```python
from build123d import *

# Parameters (mm, degrees)
SKETCH1_W                      = 203.2
SKETCH1_H                      = 203.2
BOSS_EXTRUDE1_DEPTH            = 76.2
SKETCH2_W                      = 196.85
SKETCH2_H                      = 196.85
CUT_EXTRUDE1_DEPTH             = 73.025
CUT_EXTRUDE2_REACH             = 241.623
SKETCH3_R                      = 4.7625
SKETCH3_R_2                    = 3.175
SKETCH3_W                      = 19.05
SKETCH3_H                      = 19.05
CUT_EXTRUDE2_DIRECTION_2_DEPTH = 240.623120754
CUT_EXTRUDE3_REACH             = 241.623
SKETCH4_R                      = 3.175
SKETCH4_W                      = 25.4
SKETCH4_H                      = 9.525
CUT_EXTRUDE4_REACH             = 241.623
SKETCH5_W                      = 25.4
SKETCH5_H                      = 9.525


with BuildPart() as part:
    # Sketch1 → Boss-Extrude1 (new body)
    with BuildSketch(Plane(origin=(0, 0, 0), x_dir=(1, 0, 0), z_dir=(0, 1, 0))):
        Rectangle(SKETCH1_W, SKETCH1_H)
    extrude(amount=BOSS_EXTRUDE1_DEPTH)

    # Sketch2 → Cut-Extrude1 (cut)
    with BuildSketch(Plane(origin=(0, 76.2, 0), x_dir=(1, 0, 0), z_dir=(0, 1, 0))):
        Rectangle(SKETCH2_W, SKETCH2_H)
    extrude(amount=-CUT_EXTRUDE1_DEPTH, mode=Mode.SUBTRACT)

    # Sketch3 → Cut-Extrude2 (cut, up to next)
    with BuildSketch(Plane(origin=(101.6, 0, 0), x_dir=(0, 0, -1), z_dir=(1, 0, 0)), mode=Mode.PRIVATE) as cut_extrude2_sk1:
        with Locations(Location((-69.85, 12.7, 0), (0, 0, 180))):
            Circle(SKETCH3_R)
    cut_extrude2_tool1 = extrude(cut_extrude2_sk1.sketch, amount=-CUT_EXTRUDE2_REACH, mode=Mode.PRIVATE) & part.part
    # Sketch3 → Cut-Extrude2 (cut, up to next)
    with BuildSketch(Plane(origin=(101.6, 0, 0), x_dir=(0, 0, -1), z_dir=(1, 0, 0)), mode=Mode.PRIVATE) as cut_extrude2_sk2:
        with Locations(Location((-57.15, 12.7, 0), (0, 0, 180))):
            Circle(SKETCH3_R)
    cut_extrude2_tool2 = extrude(cut_extrude2_sk2.sketch, amount=-CUT_EXTRUDE2_REACH, mode=Mode.PRIVATE) & part.part
    # Sketch3 → Cut-Extrude2 (cut, up to next)
    with BuildSketch(Plane(origin=(101.6, 0, 0), x_dir=(0, 0, -1), z_dir=(1, 0, 0)), mode=Mode.PRIVATE) as cut_extrude2_sk3:
        with Locations(Location((-44.45, 12.7, 0), (0, 0, 180))):
            Circle(SKETCH3_R)
    cut_extrude2_tool3 = extrude(cut_extrude2_sk3.sketch, amount=-CUT_EXTRUDE2_REACH, mode=Mode.PRIVATE) & part.part
    # Sketch3 → Cut-Extrude2 (cut, up to next)
    with BuildSketch(Plane(origin=(101.6, 0, 0), x_dir=(0, 0, -1), z_dir=(1, 0, 0)), mode=Mode.PRIVATE) as cut_extrude2_sk4:
        with Locations(Location((-31.75, 12.7, 0), (0, 0, 180))):
            Circle(SKETCH3_R)
    cut_extrude2_tool4 = extrude(cut_extrude2_sk4.sketch, amount=-CUT_EXTRUDE2_REACH, mode=Mode.PRIVATE) & part.part
    # Sketch3 → Cut-Extrude2 (cut, up to next)
    with BuildSketch(Plane(origin=(101.6, 0, 0), x_dir=(0, 0, -1), z_dir=(1, 0, 0)), mode=Mode.PRIVATE) as cut_extrude2_sk5:
        with Locations(Location((-88.9, 63.5, 0), (0, 0, 180))):
            Circle(SKETCH3_R_2)
    cut_extrude2_tool5 = extrude(cut_extrude2_sk5.sketch, amount=-CUT_EXTRUDE2_REACH, mode=Mode.PRIVATE) & part.part
    # Sketch3 → Cut-Extrude2 (cut, up to next)
    with BuildSketch(Plane(origin=(101.6, 0, 0), x_dir=(0, 0, -1), z_dir=(1, 0, 0)), mode=Mode.PRIVATE) as cut_extrude2_sk6:
        with Locations((22.225, 12.7)):
            Rectangle(SKETCH3_W, SKETCH3_H)
    cut_extrude2_tool6 = extrude(cut_extrude2_sk6.sketch, amount=-CUT_EXTRUDE2_REACH, mode=Mode.PRIVATE) & part.part
    add(cut_extrude2_tool1.solids().sort_by_distance((101.6, 12.7, 69.85))[0], mode=Mode.SUBTRACT)
    add(cut_extrude2_tool2.solids().sort_by_distance((101.6, 12.7, 57.15))[0], mode=Mode.SUBTRACT)
    add(cut_extrude2_tool3.solids().sort_by_distance((101.6, 12.7, 44.45))[0], mode=Mode.SUBTRACT)
    add(cut_extrude2_tool4.solids().sort_by_distance((101.6, 12.7, 31.75))[0], mode=Mode.SUBTRACT)
    add(cut_extrude2_tool5.solids().sort_by_distance((101.6, 63.5, 88.9))[0], mode=Mode.SUBTRACT)
    add(cut_extrude2_tool6.solids().sort_by_distance((101.6, 12.7, -22.225))[0], mode=Mode.SUBTRACT)

    # Sketch3 → Cut-Extrude2 direction 2 (cut)
    with BuildSketch(Plane(origin=(101.6, 0, 0), x_dir=(0, 0, -1), z_dir=(1, 0, 0))):
        with Locations(Location((-69.85, 12.7, 0), (0, 0, 180))):
            Circle(SKETCH3_R)
        with Locations(Location((-57.15, 12.7, 0), (0, 0, 180))):
            Circle(SKETCH3_R)
        with Locations(Location((-44.45, 12.7, 0), (0, 0, 180))):
            Circle(SKETCH3_R)
        with Locations(Location((-31.75, 12.7, 0), (0, 0, 180))):
            Circle(SKETCH3_R)
        with Locations(Location((-88.9, 63.5, 0), (0, 0, 180))):
            Circle(SKETCH3_R_2)
        with Locations((22.225, 12.7)):
            Rectangle(SKETCH3_W, SKETCH3_H)
    extrude(amount=CUT_EXTRUDE2_DIRECTION_2_DEPTH, mode=Mode.SUBTRACT)

    # Sketch4 → Cut-Extrude3 (cut, up to next)
    with BuildSketch(Plane(origin=(0, 0, -101.6), x_dir=(-1, 0, 0), z_dir=(0, 0, -1)), mode=Mode.PRIVATE) as cut_extrude3_sk1:
        with Locations((0, 38.1)):
            Circle(SKETCH4_R)
    cut_extrude3_tool1 = extrude(cut_extrude3_sk1.sketch, amount=-CUT_EXTRUDE3_REACH, mode=Mode.PRIVATE) & part.part
    # Sketch4 → Cut-Extrude3 (cut, up to next)
    with BuildSketch(Plane(origin=(0, 0, -101.6), x_dir=(-1, 0, 0), z_dir=(0, 0, -1)), mode=Mode.PRIVATE) as cut_extrude3_sk2:
        with Locations((50.8, 38.1)):
            Rectangle(SKETCH4_W, SKETCH4_H)
    cut_extrude3_tool2 = extrude(cut_extrude3_sk2.sketch, amount=-CUT_EXTRUDE3_REACH, mode=Mode.PRIVATE) & part.part
    add(cut_extrude3_tool1.solids().sort_by_distance((0, 38.1, -101.6))[0], mode=Mode.SUBTRACT)
    add(cut_extrude3_tool2.solids().sort_by_distance((-50.8, 38.1, -101.6))[0], mode=Mode.SUBTRACT)

    # Sketch5 → Cut-Extrude4 (cut, up to next)
    with BuildSketch(Plane.ZY.offset(101.6), mode=Mode.PRIVATE) as cut_extrude4_sk1:
        with Locations((-15.875, 38.1)):
            Rectangle(SKETCH5_W, SKETCH5_H)
    cut_extrude4_tool1 = extrude(cut_extrude4_sk1.sketch, amount=-CUT_EXTRUDE4_REACH, mode=Mode.PRIVATE) & part.part
    # Sketch5 → Cut-Extrude4 (cut, up to next)
    with BuildSketch(Plane.ZY.offset(101.6), mode=Mode.PRIVATE) as cut_extrude4_sk2:
        with Locations((-47.625, 38.1)):
            Rectangle(SKETCH5_W, SKETCH5_H)
    cut_extrude4_tool2 = extrude(cut_extrude4_sk2.sketch, amount=-CUT_EXTRUDE4_REACH, mode=Mode.PRIVATE) & part.part
    # Sketch5 → Cut-Extrude4 (cut, up to next)
    with BuildSketch(Plane.ZY.offset(101.6), mode=Mode.PRIVATE) as cut_extrude4_sk3:
        with Locations((47.625, 38.1)):
            Rectangle(SKETCH5_W, SKETCH5_H)
    cut_extrude4_tool3 = extrude(cut_extrude4_sk3.sketch, amount=-CUT_EXTRUDE4_REACH, mode=Mode.PRIVATE) & part.part
    # Sketch5 → Cut-Extrude4 (cut, up to next)
    with BuildSketch(Plane.ZY.offset(101.6), mode=Mode.PRIVATE) as cut_extrude4_sk4:
        with Locations((15.875, 38.1)):
            Rectangle(SKETCH5_W, SKETCH5_H)
    cut_extrude4_tool4 = extrude(cut_extrude4_sk4.sketch, amount=-CUT_EXTRUDE4_REACH, mode=Mode.PRIVATE) & part.part
    add(cut_extrude4_tool1.solids().sort_by_distance((-101.6, 38.1, -15.875))[0], mode=Mode.SUBTRACT)
    add(cut_extrude4_tool2.solids().sort_by_distance((-101.6, 38.1, -47.625))[0], mode=Mode.SUBTRACT)
    add(cut_extrude4_tool3.solids().sort_by_distance((-101.6, 38.1, 47.625))[0], mode=Mode.SUBTRACT)
    add(cut_extrude4_tool4.solids().sort_by_distance((-101.6, 38.1, 15.875))[0], mode=Mode.SUBTRACT)


solid = part.part
```
Can you work these out from the model? Positions are in its coordinate system, mm. A direction names the side the tool comes from. Give positions to 0.01 mm unless a question says otherwise; leave off trailing zeros. Write each loop counter-clockwise with the first axis right and the second up, starting at its lowest first coordinate (ties: lowest second). Pieces come first, ordered by that corner, then holes. Notation, with made-up numbers: (88.25, 24.25) -> (147.25, 24.25) arc R23 ccw to (147.25, 49.25) -> close; hole circle Ø5 at (12.5, 23.25). An arc over 180 degrees is marked (long way). Write item = value, one per line.
(1) Suppose I cut it at D-D on z = 69.85. Write out the boundary of the cut face in (x, y) (1 decimal), then the cut area to 3 significant figures.
Worked out:
outline = (-101.6, 0) -> (101.6, 0) -> (101.6, 7.9) -> (98.4, 7.9) -> (98.4, 3.2) -> (-98.4, 3.2) -> (-98.4, 76.2) -> (-101.6, 76.2) -> close; (98.4, 17.5) -> (101.6, 17.5) -> (101.6, 76.2) -> (98.4, 76.2) -> close
area = 1,080 mm^2
(2) Thinking about a two-plate mould opening in X: for faces 1 (the face through (100, 11.3, 36.3)), 2 (the face through (98.425, 40, 1)), 3 (the face through (-101.6, 38, 1)), which applies, released by +X, released by -X, zero draft, split by the parting line, or undercut?
Worked out:
face_1 = zero draft
face_2 = undercut
face_3 = released by -X
(3) I need wall thicknesses on probe 1 along Z at (x, y) = (100.9, 12.7); probe 2 along Z at (x, y) = (-46, 29.5) (3 decimals). Which ranges of each line are inside material? Lowest first, please. Write a range as from..to.
Worked out:
probe_1 = -101.6..-31.75, -12.7..26.99, 36.51..39.69, 49.21..52.39, 61.91..65.09, 74.61..101.6
probe_2 = -101.6..-98.425, 98.425..101.6
(4) Suppose I cut it at C-C on x = -59. Write out the boundary of the cut face in (y, z) (1 decimal).
Worked out:
outline = (0, -101.6) -> (33.3, -101.6) -> (33.3, -98.4) -> (3.2, -98.4) -> (3.2, 98.4) -> (76.2, 98.4) -> (76.2, 101.6) -> (0, 101.6) -> close; (42.9, -101.6) -> (76.2, -101.6) -> (76.2, -98.4) -> (42.9, -98.4) -> close
(5) I'm going to push flat-ended pins straight in: P1, Ø5.5, axis at y = 12.7, z = 57.15, coming from the +X side (3 decimals); P2, Ø1, axis at x = -63, z = 77, coming from the +Y side (3 decimals); P3, Ø1.5, axis at y = 35, z = 5, coming from the -X side (3 decimals). Where does each tip first touch, or does it pass through?
Worked out:
P1 = -98.425
P2 = 3.175
P3 = 98.425
(6) Suppose I cut it at A-A on z = 44.45. Write out the boundary of the cut face in (x, y) (1 decimal).
Worked out:
outline = (-101.6, 0) -> (101.6, 0) -> (101.6, 7.9) -> (98.4, 7.9) -> (98.4, 3.2) -> (-98.4, 3.2) -> (-98.4, 33.3) -> (-101.6, 33.3) -> close; (-101.6, 42.9) -> (-98.4, 42.9) -> (-98.4, 76.2) -> (-101.6, 76.2) -> close; (98.4, 17.5) -> (101.6, 17.5) -> (101.6, 76.2) -> (98.4, 76.2) -> close
(7) Suppose I cut it at B-B on y = 12.7. Count the separate pieces of the cut face and the enclosed holes in it, then the cut area to 3 significant figures.
Worked out:
separate_pieces = 5
enclosed_holes = 0
area = 2,360 mm^2
(8) For faces 4 (the face through (100.035, 8.684, 72.41)), 5 (the face through (-98.425, 40, 1)), 6 (the face through (0.69, 35, -100.03)), which set-ups out of +Z, -Z, +X, -X, +Y, -Y let a thin tool reach every point of the face, with its end or its side?
Worked out:
face_4 = +X
face_5 = +Y
face_6 = -Z
